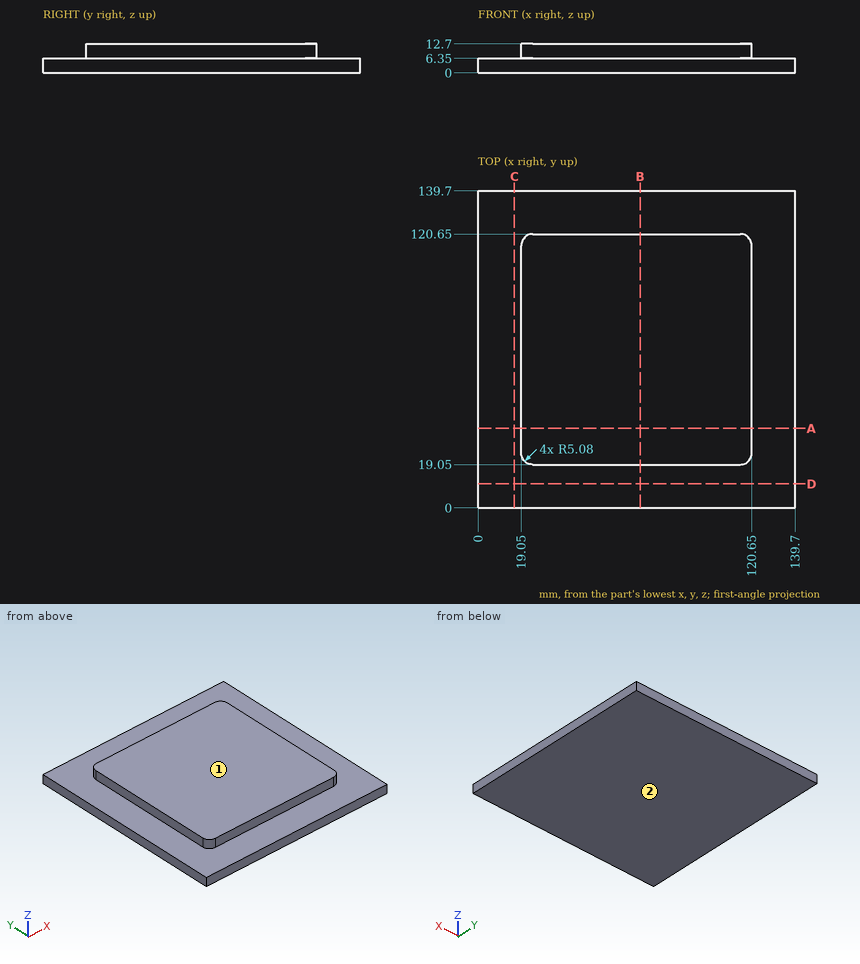
The figure shows three views and two pictorial views of one solid part (mm, origin at its lowest corner). Answer the questions. Coordinates: 2 decimals unless noted, no trailing zeros. Loops run counter-clockwise (first coordinate to the right, second up) from the corner with the lowest first, then second, coordinate; pieces in that order, holes last. Notation, with made-up numbers: (25, 19.25) -> (78, 19.25) arc R25 ccw to (78, 54.25) -> close; hole circle Ø7 at (40, 23.25). An arc over 180 degrees is marked (long way). Write item = value, one per line. Start each with the question number.
1) A cutting plane is placed at A-A (y = 35). Give the vertices of the cut face in (x, z), then the cut area to 3 significant figures.
2) Given pin 1 Ø1 at (y, z) = (14.5, 6.5) entering from -X; pin 2 Ø1.9 at (y, z) = (65, 11) entering from -X; pin 3 Ø1 at (x, z) = (72.5, 7) entering from +Y; pin 4 Ø7 at (x, z) = (61.5, 10) entering from -Y, each flat-ended and moving along its own axis, determine where each tip first touches the part or whether it passes through.
3) Straight lines are drawn through the part: line 1 (X direction, y = 39, z = 6.5); line 2 (Z direction, x = 55, y = 7). For each, find the intervals that lie inside material, in ascending order. Write a range as from..to.
4) The mould has two halves that part along Z. Classify the marked faces 1 and 2: released by +Z, released by -Z, zero draft, split by the parting line, or undercut.
5) A cutting plane is placed at C-C (x = 16). Give the vertices of the cut face in (y, z), then the cut area to 3 significant figures.
Responses:
q1.outline = (0, 0) -> (139.7, 0) -> (139.7, 6.35) -> (120.65, 6.35) -> (120.65, 12.7) -> (19.05, 12.7) -> (19.05, 6.35) -> (0, 6.35) -> close
q1.area = 1,530 mm²
q2.pin_1 = 0
q2.pin_2 = 19.05
q2.pin_3 = 120.65
q2.pin_4 = 19.05
q3.line_1 = 19.05..120.65
q3.line_2 = 0..6.35
q4.face_1 = released by +Z
q4.face_2 = released by -Z
q5.outline = (0, 0) -> (139.7, 0) -> (139.7, 6.35) -> (0, 6.35) -> close
q5.area = 887 mm²
